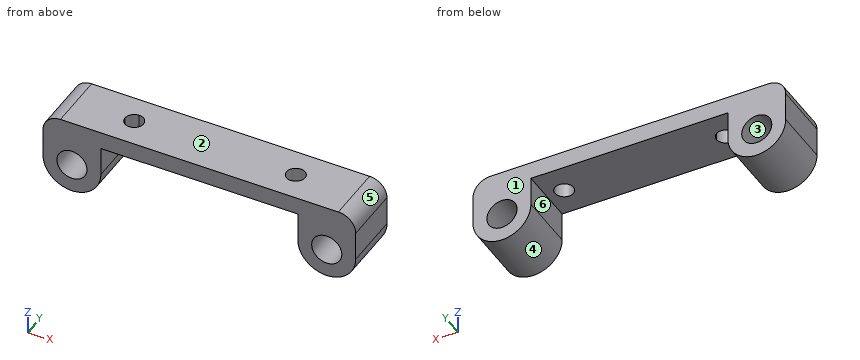
from build123d import *

# Parameters (mm, degrees)
EXTRUDE_1_DEPTH = 3
SKETCH_2_R      = 5
SKETCH_2_R_2    = 2.6
EXTRUDE_2_DEPTH = 10
FILLET_1_R      = 3


with BuildPart() as part:
    # 草图1 → 凸台-拉伸1 (new body)
    with BuildSketch(Plane.XY):
        with BuildLine():
            Line((0, 5), (-13.95, 5))
            Line((-13.95, 5), (-13.95, 1.6))
            ThreePointArc((-13.95, 1.6), (-12.81862915, 1.13137085), (-12.35, 0))
            Line((-12.35, 0), (0, 0))
            Line((0, 0), (0, 5))
        make_face()
        with BuildLine():
            Line((-27, 5), (-27, 0))
            Line((-27, 0), (-17, 0))
            Line((-17, 0), (-15.55, 0))
            ThreePointArc((-15.55, 0), (-15.08137085, 1.13137085), (-13.95, 1.6))
            Line((-13.95, 1.6), (-13.95, 5))
            Line((-13.95, 5), (-27, 5))
        make_face()
        with BuildLine():
            Line((-17, 0), (-27, 0))
            Line((-27, 0), (-27, -5))
            Line((-27, -5), (27, -5))
            Line((27, -5), (27, 0))
            Line((27, 0), (17, 0))
            Line((17, 0), (15.55, 0))
            ThreePointArc((15.55, 0), (13.95, -1.6), (12.35, 0))
            Line((12.35, 0), (0, 0))
            Line((0, 0), (-12.35, 0))
            ThreePointArc((-12.35, 0), (-13.95, -1.6), (-15.55, 0))
            Line((-15.55, 0), (-17, 0))
        make_face()
        with BuildLine():
            Line((17, 0), (27, 0))
            Line((27, 0), (27, 5))
            Line((27, 5), (0, 5))
            Line((0, 5), (0, 0))
            Line((0, 0), (12.35, 0))
            ThreePointArc((12.35, 0), (13.95, 1.6), (15.55, 0))
            Line((15.55, 0), (17, 0))
        make_face()
    extrude(amount=EXTRUDE_1_DEPTH)

    # 草图2 → 凸台-拉伸2 (add, through all)
    # profile 1 of 6: a face of its own
    with BuildSketch(Plane(origin=(0, 5, 0), x_dir=(1, 0, 0), z_dir=(0, 1, 0))):
        with Locations((-22, 5)):
            Circle(SKETCH_2_R)
        with Locations(Location((-22, 5, 0), (0, 0, 270))):
            Circle(SKETCH_2_R_2, mode=Mode.SUBTRACT)
    # profile 2 of 6: a face of its own
    with BuildSketch(Plane(origin=(0, 5, 0), x_dir=(1, 0, 0), z_dir=(0, 1, 0))):
        with BuildLine():
            Line((-17, 0), (-17, 5))
            ThreePointArc((-17, 5), (-18.464466102, 1.464466086), (-22.000000023, 0))
            Line((-22.000000023, 0), (-17, 0))
        make_face()
    # profile 3 of 6: a face of its own
    with BuildSketch(Plane(origin=(0, 5, 0), x_dir=(1, 0, 0), z_dir=(0, 1, 0))):
        with BuildLine():
            ThreePointArc((-22.000000023, 0), (-25.535533914, 1.464466102), (-27, 5))
            Line((-27, 5), (-27, 0))
            Line((-27, 0), (-22.000000023, 0))
        make_face()
    # profile 4 of 6: a face of its own
    with BuildSketch(Plane(origin=(0, 5, 0), x_dir=(1, 0, 0), z_dir=(0, 1, 0))):
        with BuildLine():
            Line((17, 5), (17, 0))
            Line((17, 0), (22, 0))
            ThreePointArc((22, 0), (18.464466094, 1.464466094), (17, 5))
        make_face()
    # profile 5 of 6: a face of its own
    with BuildSketch(Plane(origin=(0, 5, 0), x_dir=(1, 0, 0), z_dir=(0, 1, 0))):
        with Locations((22, 5)):
            Circle(SKETCH_2_R)
        with Locations(Location((22, 5, 0), (0, 0, 270))):
            Circle(SKETCH_2_R_2, mode=Mode.SUBTRACT)
    # profile 6 of 6: a face of its own
    with BuildSketch(Plane(origin=(0, 5, 0), x_dir=(1, 0, 0), z_dir=(0, 1, 0))):
        with BuildLine():
            ThreePointArc((27, 5), (25.535533906, 1.464466094), (22, 0))
            Line((22, 0), (27, 0))
            Line((27, 0), (27, 5))
        make_face()
    extrude(amount=-EXTRUDE_2_DEPTH)

    # 圆角1
    fillet_1_edges = [part.edges().sort_by_distance(p)[0] for p in [
        (27, 0, 3),
        (-27, 0, 3),
    ]]
    fillet(fillet_1_edges, radius=FILLET_1_R)


solid = part.part
Can you work these out from the model? Positions are in its coordinate system, mm. Face numbers are marked on the shaded views. A direction names the side the tool comes from. Round coordinates to 2 decimals unless told otherwise and drop trailing zeros. Write each loop counter-clockwise with the first axis right and the second up, starting at its lowest first coordinate (ties: lowest second). Pieces come first, ordered by that corner, then holes. Notation, with made-up numbers: (15, -10) - (19, -10) arc R28 ccw to (19, 29) - close; hole circle Ø10 at (18, -11). An arc over 180 degrees is marked (long way). Write each question's results on one line, items separated by ' | '. Start each with the question number.
1) Suppose I cut it at A-A (x = -22). List the corners of the cut face in (y, z) for me, and give its area (3 significant figures).
2) We'd pull the mould along Z, two halves only. Please class the marked faces 1, 2, 3 and 4: released by +Z, released by -Z, zero draft, split by the parting line, or undercut.
3) For pin 1 Ø3 at (x, y) = (6.5, -0.5) entering from -Z, with a flat end and sliding along its axis, tell me the tip position at first contact or that it passes through.
4) Suppose I cut it at D-D (z = -6.5). List the corners of the cut face in (x, y) for me.
5) Please list where these lines run through material, in increasing order: line 1 (X direction, y = -0.25, z = -5); line 2 (X direction, y = -3.25, z = -2.25); line 3 (X direction, y = -0.5, z = 2).
6) Which directions (+Z, -Z, +X, -X, +Y, -Y) give clear straight access to the entire face, cutting with the end or side of a thin tool? Please do the marked faces 5 and 6.
7) Suppose I cut it at B-B (y = -4.25). List the corners of the cut face in (x, z) for me.
8) Suppose I cut it at C-C (z = -1). List the corners of the cut face in (x, y) for me.
Here are the results:
1) outline: (-5, -10) - (5, -10) - (5, -7.6) - (-5, -7.6) - close; (-5, -2.4) - (5, -2.4) - (5, 3) - (-5, 3) - close | area: 78.0 mm2
2) face 1: zero draft | face 2: released by +Z | face 3: undercut | face 4: released by -Z
3) pin 1: stops at z = 0
4) outline: (-26.77, -5) - (-24.12, -5) - (-24.12, 5) - (-26.77, 5) - close; (-19.88, -5) - (-17.23, -5) - (-17.23, 5) - (-19.88, 5) - close; (17.23, -5) - (19.88, -5) - (19.88, 5) - (17.23, 5) - close; (24.12, -5) - (26.77, -5) - (26.77, 5) - (24.12, 5) - close
5) line 1: x = -27 to -24.6, -19.4 to -17, 17 to 19.4, 24.6 to 27 | line 2: x = -27 to -17, 17 to 27 | line 3: x = -26.24 to -15.47, -12.43 to 12.43, 15.47 to 26.24
6) face 5: +Z, +X, +Y, -Y | face 6: -Z, +Y, -Y
7) outline: (-27, -5) arc R5 ccw to (-17, -5) - (-17, 0) - (17, 0) - (17, -5) arc R5 ccw to (27, -5) - (27, 0) arc R3 ccw to (24, 3) - (-24, 3) arc R3 ccw to (-27, 0) - close; hole circle Ø5.2 at (-22, -5); hole circle Ø5.2 at (22, -5)
8) outline: (-27, -5) - (-17, -5) - (-17, 5) - (-27, 5) - close; (17, -5) - (27, -5) - (27, 5) - (17, 5) - close
